from build123d import *

# Parameters (mm, degrees)
F0_W      = 12.7
F0_H      = 25.4
F1_DEPTH  = 101.6
F2_W      = 82.55
F2_H      = 25.4
F3_DEPTH  = 69.851
F4_W      = 44.45
F4_H      = 50.8
F4_H_2    = 25.4
F5_DEPTH  = 25.4
F6_R      = 5.08
F7_R      = 6.35
F7_R_2    = 3.302
F8_DEPTH  = 69.85
F9_R      = 3.302
F10_DEPTH = 69.851
F12_DEPTH = 6.35
F13_R     = 4.8460610966
F13_R_2   = 3.048
F14_DEPTH = 19.05
F15_R     = 3.048
F16_DEPTH = 69.851
F18_R     = 7.62
F19_DEPTH = 19.05
F20_R     = 7.62
F21_DEPTH = 19.05


# Not quite as in the source:
# - two fillets or chamfers of one size are made in one step
# - a feature names something its author has since deleted; it is built from what else it names


with BuildPart() as f1:
    # F0 (on Front) → F1 (new body)
    with BuildSketch(Plane.XZ):
        Polygon((34.925, -6.35), (34.925, 6.35), (22.225, 6.35), (-22.225, 6.35), (-34.925, 6.35), (-34.925, -6.35), align=None)
        with Locations((28.575, 19.05)):
            Rectangle(F0_W, F0_H)
        with Locations((-28.575, 19.05)):
            Rectangle(F0_W, F0_H)
    extrude(amount=F1_DEPTH)

    # F2 (on face) → F3 (cut, through all)
    with BuildSketch(Plane.YZ.offset(34.925)):
        with Locations((-41.275, 19.05)):
            Rectangle(F2_W, F2_H)
        with BuildLine():
            ThreePointArc((-86.36, 19.05), (-87.8478975516, 22.6421024484), (-91.44, 24.13))
            Line((-91.44, 24.13), (-91.44, 19.05))
            Line((-91.44, 19.05), (-96.52, 19.05))
            ThreePointArc((-96.52, 19.05), (-91.44, 13.97), (-86.36, 19.05))
        make_face()
        with BuildLine():
            Line((-91.44, 19.05), (-91.44, 24.13))
            ThreePointArc((-91.44, 24.13), (-95.0321024484, 22.6421024484), (-96.52, 19.05))
            Line((-96.52, 19.05), (-91.44, 19.05))
        make_face()
    extrude(amount=-F3_DEPTH, mode=Mode.SUBTRACT)

    # F4 (on face) → F5 (cut)
    with BuildSketch(Plane.XY.offset(6.35)):
        with Locations((0, -50.8)):
            Rectangle(F4_W, F4_H)
        with Locations((0, -88.9)):
            Rectangle(F4_W, F4_H_2)
    extrude(amount=-F5_DEPTH, mode=Mode.SUBTRACT)

    # F6
    f6_edges = [f1.edges().sort_by_distance(p)[0] for p in [
        (-28.575, -101.6, 31.75),
        (-28.575, -82.55, 31.75),
        (28.575, -101.6, 31.75),
        (28.575, -82.55, 31.75),
        (22.225, -25.4, 0),
        (-22.225, -25.4, 0),
    ]]
    fillet(f6_edges, radius=F6_R)

    # F7 (on face) → F8 (join, through all)
    with BuildSketch(Plane.YZ.offset(34.925)):
        Circle(F7_R)
        Circle(F7_R_2, mode=Mode.SUBTRACT)
    extrude(amount=-F8_DEPTH)

    # F9 (on face) → F10 (cut, through all)
    with BuildSketch(Plane.YZ.offset(34.925)):
        Circle(F9_R)
    extrude(amount=-F10_DEPTH, mode=Mode.SUBTRACT)

    # F11 (on Front) → F12 (cut, symmetric)
    with BuildSketch(Plane.XZ):
        Polygon((-9.525, -12.2059704736), (-9.525, 0), (-9.525, 12.2059704736), (-28.575, 12.2059704736), (-28.575, -12.2059704736), align=None)
        Polygon((9.525, 10.1526007056), (9.525, 0), (9.525, -10.1526007056), (28.575, -10.1526007056), (28.575, 10.1526007056), align=None)
    extrude(amount=F12_DEPTH, both=True, mode=Mode.SUBTRACT)

    # F13 (on face) → F14 (join, through all)
    with BuildSketch(Plane.YZ.offset(9.525)):
        Circle(F13_R)
        Circle(F13_R_2, mode=Mode.SUBTRACT)
    extrude(amount=-F14_DEPTH)

    # F15 (on face) → F16 (cut, through all)
    with BuildSketch(Plane.YZ.offset(34.925)):
        with Locations((-25.4, 0)):
            Circle(F15_R)
    extrude(amount=-F16_DEPTH, mode=Mode.SUBTRACT)

    # F18 (on face) → F19 (cut, through all)
    with BuildSketch(Plane.YZ.offset(9.525)):
        Circle(F18_R)
    extrude(amount=F19_DEPTH, mode=Mode.SUBTRACT)

    # F20 (on face) → F21 (cut, through all)
    with BuildSketch(Plane(origin=(-9.525, 0, 0), x_dir=(0, -1, 0), z_dir=(-1, 0, 0))):
        Circle(F20_R)
    extrude(amount=F21_DEPTH, mode=Mode.SUBTRACT)


solid = f1.part
CAD build for the part. Positions are in the model's coordinates, mm. A direction names the side the tool comes from. Coordinates: 2 decimals unless noted, no trailing zeros. Write each loop counter-clockwise with the first axis right and the second up, starting at its lowest first coordinate (ties: lowest second). Pieces come first, ordered by that corner, then holes. Notation, with made-up numbers: (-25.75, 30.25) - (5.25, 30.25) arc R17 cw to (5.25, 59.25) - close; hole circle Ø3 at (68.25, 86.25). An arc over 180 degrees is marked (long way). Use a Markdown table: item, result. Add a question column.
Item 1: Band-saw the part on D-D, the plane z = 0. Give the number of separate pieces and of enclosed holes in the cut face, and give its area (3 significant figures).
Item 2: Band-saw the part on C-C, the plane y = -63. Give the cut face in (x, z) (3 decimals).
Item 3: Band-saw the part on B-B, the plane x = -25. Give the cut face in (y, z).
Item 4: Mould opens along Z. For faces 6 (the face through (-19, -6.35, 5)), 7 (the face through (18.92, -7.62, 0.06)), 8 (the face through (28.486, -84.078, 30.301)) say: pulls with the +Z half, pulls with the -Z half, needs draft (parallel to the pull), parting line crosses it, or undercut.
Item 5: Flat gauge pins, fed straight in: pin 1 (1 mm diameter, centred on x = -23, y = -38, fed in from +Z); pin 2 (1.7 mm diameter, centred on x = 19.5, z = 5.5, fed in from +Y); pin 3 (4 mm diameter, centred on x = 25.5, z = 15.5, fed in from +Y). Where does each tip first touch, or does it go through?
Item 6: 3-axis set-ups, long thin cutter, end or side, ignore diameter. For faces 1 (the face through (-29, -101.6, 10)), 2 (the face through (19, -6.35, 5)), 3 (the face through (-31.71, 1.26, 3.05)), 4 (the face through (-28, -82.55, 16)), 5 (the face through (0, -25.4, -5)): which of +Z, -Z, +X, -X, +Y, -Y reach the whole face in a straight line?
Item 7: Drill centre lines: L1, parallel to Y at x = -33.25, z = 0; L2, parallel to X at y = 2, z = 5.5 (3 decimals); L3, parallel to Z at x = 0.25, y = 0. Where is each one in solid material? Low to high. Write a range as from..to.
Item 8: Band-saw the part on A-A, the plane z = 8. Give the cut face in (x, y) (3 decimals).
Numbers:
| question | item | result |
|---|---|---|
| 1 | separate pieces | 6 |
| 1 | enclosed holes | 0 |
| 1 | area | 3,130 mm2 |
| 2 | outline | (-34.925, -6.35) - (-22.225, -6.35) - (-22.225, 6.35) - (-34.925, 6.35) - close; (22.225, -6.35) - (34.925, -6.35) - (34.925, 6.35) - (22.225, 6.35) - close |
| 3 | outline | (-101.6, -6.35) - (-6.35, -6.35) - (-6.35, -4.21) arc R7.62 cw to (-6.35, 4.21) - (-6.35, 6.35) - (-82.55, 6.35) - (-82.55, 26.67) arc R5.08 ccw to (-87.63, 31.75) - (-96.52, 31.75) arc R5.08 ccw to (-101.6, 26.67) - close; hole circle Ø10.16 at (-91.44, 19.05); hole circle Ø6.1 at (-25.4, 0) |
| 4 | face 6 | needs draft |
| 4 | face 7 | undercut |
| 4 | face 8 | pulls with the +Z half |
| 5 | pin 1 | z = 6.35 |
| 5 | pin 2 | y = -6.35 |
| 5 | pin 3 | y = -82.55 |
| 6 | face 1 | +Z, -Z, +X, -X, -Y |
| 6 | face 2 | +Z, -Z, +Y |
| 6 | face 3 | -X |
| 6 | face 4 | +Z, +X, -X, +Y |
| 6 | face 5 | +Z, -Z, -Y |
| 7 | L1 | -101.6..-28.45, -22.35..-3.3, 3.3..6.35 |
| 7 | L2 | -34.925..-28.575, -9.525..9.525, 28.575..34.925 |
| 7 | L3 | -6.35..-3.05, 3.05..6.35 |
| 8 | outline | (-34.925, -101.6) - (-22.225, -101.6) - (-22.225, -82.55) - (-34.925, -82.55) - close; (22.225, -101.6) - (34.925, -101.6) - (34.925, -82.55) - (22.225, -82.55) - close |
